Model file for the job. Use its own axes, mm. Round coordinates to 2 decimals unless told otherwise and drop trailing zeros. Loops run counter-clockwise (first coordinate to the right, second up) from the corner with the lowest first, then second, coordinate; pieces in that order, holes last. Notation, with made-up numbers: (27.5, 42.25) - (32.5, 42.25) arc R25 ccw to (32.5, 55.25) - close; hole circle Ø7 at (7, 81). An arc over 180 degrees is marked (long way). Use one line per item in the form item = value.
from build123d import *

# Parameters (mm, degrees)
SKETCH1_W           = 102
SKETCH1_H           = 12
SKETCH1_R           = 1.6
BOSS_EXTRUDE1_DEPTH = 3
FILLET1_R           = 4


with BuildPart() as part:
    # Sketch1 → Boss-Extrude1 (new, symmetric)
    with BuildSketch(Plane(origin=(0, 0, 0), x_dir=(1, 0, 0), z_dir=(0, 1, 0))):
        Rectangle(SKETCH1_W, SKETCH1_H)
        with Locations(Location((-45, 0, 0), (0, 0, 270))):
            Circle(SKETCH1_R, mode=Mode.SUBTRACT)
        with Locations(Location((-20.5, 0, 0), (0, 0, 270))):
            Circle(SKETCH1_R, mode=Mode.SUBTRACT)
        with Locations(Location((20.5, 0, 0), (0, 0, 270))):
            Circle(SKETCH1_R, mode=Mode.SUBTRACT)
        with Locations(Location((45, 0, 0), (0, 0, 270))):
            Circle(SKETCH1_R, mode=Mode.SUBTRACT)
    extrude(amount=BOSS_EXTRUDE1_DEPTH, both=True)

    # Fillet1
    fillet1_edges = [part.edges().sort_by_distance(p)[0] for p in [
        (51, 0, 6),
        (-51, 0, 6),
        (-51, 0, -6),
        (51, 0, -6),
    ]]
    fillet(fillet1_edges, radius=FILLET1_R)


solid = part.part
1. Cut at D-D, the plane z = 5. Give the cut face in (x, y), plus the area to 3 significant figures.
Geometry check:
outline = (-49.65, -3) - (49.65, -3) - (49.65, 3) - (-49.65, 3) - close
area = 596 mm^2
2. Cut at B-B, the plane z = 0. Give the cut face in (x, y), plus the area to 3 significant figures.
Geometry check:
outline = (-51, -3) - (-46.6, -3) - (-46.6, 3) - (-51, 3) - close; (-43.4, -3) - (-22.1, -3) - (-22.1, 3) - (-43.4, 3) - close; (-18.9, -3) - (18.9, -3) - (18.9, 3) - (-18.9, 3) - close; (22.1, -3) - (43.4, -3) - (43.4, 3) - (22.1, 3) - close; (46.6, -3) - (51, -3) - (51, 3) - (46.6, 3) - close
area = 535 mm^2
3. Cut at C-C, the plane x = -45. Give the cut face in (y, z).
Geometry check:
outline = (-3, -6) - (3, -6) - (3, -1.6) - (-3, -1.6) - close; (-3, 1.6) - (3, 1.6) - (3, 6) - (-3, 6) - close
4. Wall check: probe 1 along X at (y, z) = (0, 0); probe 2 along X at (y, z) = (0.2, -0.5); probe 3 along X at (y, z) = (-1.15, -5). Give the ranges that are in metal, low to high.
Geometry check:
probe_1 = -51 to -46.6, -43.4 to -22.1, -18.9 to 18.9, 22.1 to 43.4, 46.6 to 51
probe_2 = -51 to -46.52, -43.48 to -22.02, -18.98 to 18.98, 22.02 to 43.48, 46.52 to 51
probe_3 = -49.65 to 49.65
5. Cut at A-A, the plane y = 1.65. Give the cut face in (x, z), plus the area to 3 significant figures.
Geometry check:
outline = (-51, -2) arc R4 ccw to (-47, -6) - (47, -6) arc R4 ccw to (51, -2) - (51, 2) arc R4 ccw to (47, 6) - (-47, 6) arc R4 ccw to (-51, 2) - close; hole circle Ø3.2 at (-45, 0); hole circle Ø3.2 at (-20.5, 0); hole circle Ø3.2 at (20.5, 0); hole circle Ø3.2 at (45, 0)
area = 1,180 mm^2
6. Flat gauge pins, fed straight in: pin 1 (2.5 mm diameter, centred on x = -20.5, z = 0, fed in from -Y) (3 decimals); pin 2 (4 mm diameter, centred on x = 20.5, z = 0, fed in from -Y). Where does each tip first touch, or does it go through?
Geometry check:
pin_1 = through
pin_2 = -3
7. Pull direction Z, two halves, no side cores. Call faces 1 (the flat face through (-1, 0, 6)), 2 (the flat face through (-1, 0, -6)), 3 (the cylindrical face through (43.58, -0.04, 0.74)), 4 (the flat face through (51, 0, 0)): +Z half, -Z half, draft (parallel to the pull), parting line (faces both ways), or undercut.
Geometry check:
face_1 = +Z half
face_2 = -Z half
face_3 = undercut
face_4 = draft
